```python
from build123d import *

# Parameters (mm, degrees)
SKETCH1_W           = 254
SKETCH1_H           = 60.071
BOSS_EXTRUDE1_DEPTH = 1.778
CUT_EXTRUDE2_DEPTH  = 2.778
LPATTERN1_COUNT     = 9
LPATTERN1_PITCH     = 19.05


with BuildPart() as part:
    # Sketch1 → Boss-Extrude1 (new body)
    with BuildSketch(Plane.XY):
        with Locations((127, 30.0355)):
            Rectangle(SKETCH1_W, SKETCH1_H)
    extrude(amount=BOSS_EXTRUDE1_DEPTH)

    # Sketch1<3> → Cut-Extrude2 (cut, through all)
    with BuildSketch(Plane.XY):
        with BuildLine():
            Line((46.863, 32.359981663), (46.863, 27.711018337))
            ThreePointArc((46.863, 27.711018337), (50.8, 25.4635), (54.737, 27.711018337))
            Line((54.737, 27.711018337), (54.737, 32.359981663))
            ThreePointArc((54.737, 32.359981663), (50.8, 34.6075), (46.863, 32.359981663))
        make_face()
    cut_extrude2 = extrude(amount=CUT_EXTRUDE2_DEPTH, mode=Mode.SUBTRACT)

    # LPattern1: Cut-Extrude2 ×9
    with Locations(*[(i * LPATTERN1_PITCH, 0, 0) for i in range(1, LPATTERN1_COUNT)]):
        add(cut_extrude2, mode=Mode.SUBTRACT)


solid = part.part
```
Here's how the part is built. I have some questions about the finished solid (model axes, mm). Give positions to 0.01 mm unless a question says otherwise; leave off trailing zeros. Loops run counter-clockwise (first coordinate to the right, second up) from the corner with the lowest first, then second, coordinate; pieces in that order, holes last. Notation, with made-up numbers: M -24.75,61.25 L -18.75,61.25 A12 ccw -18.75,83.25 Z; hole C 40.5,62 d8. An arc over 180 degrees is marked long. Put each result on its own line as item: value. Start each with the question number.
(1) I want a section at A-A on x = 184. Please give me the cut outline in (y, z).
(2) I want a section at C-C on x = 109. Please give me the cut outline in (y, z).
(3) I need wall thicknesses on line 1 along Y through (x, z) = (69.5, 0.8); line 2 along Y through (x, z) = (200, 0.85). Which ranges of each line are inside material? Lowest first, please. Write a range as [from, to].
(4) I want a section at B-B on z = 0.6. State how many separate pieces and enclosed holes the cut face has, then the cut area to 3 significant figures.
Answer block:
1. outline: M 0,0 L 25.47,0 L 25.47,1.78 L 0,1.78 Z; M 34.61,0 L 60.07,0 L 60.07,1.78 L 34.61,1.78 Z
2. outline: M 0,0 L 25.59,0 L 25.59,1.78 L 0,1.78 Z; M 34.49,0 L 60.07,0 L 60.07,1.78 L 34.49,1.78 Z
3. line 1: [0, 25.48], [34.59, 60.07]
3. line 2: [0, 26.77], [33.3, 60.07]
4. separate pieces: 1
4. enclosed holes: 9
4. area: 14,700 mm^2
